The listing builds one solid part. Answer for the finished solid, in the listing's coordinates (mm). Face numbers are marked on the shaded views. A direction names the side the tool comes from. Coordinates: 2 decimals unless noted, no trailing zeros. Order: outer loops, then holes, each group sorted by start corner. A loop starts at its lowest first (then second) coordinate and runs counter-clockwise, first axis right, second up. Notation, with made-up numbers: (-4.5, -17) - (21.5, -17) arc R19 ccw to (21.5, -11) - close; hole circle Ø9 at (-26.5, 15.5). An arc over 180 degrees is marked (long way). Use one line per item in the form item = value. Start each with the question number.
Item 1: Each of these flat-tipped pins is pushed along its axis until it touches: pin 1 Ø4 at (x, y) = (0, 0) entering from +Z; pin 2 Ø4 at (x, y) = (-29, 34) entering from +Z; pin 3 Ø8 at (x, z) = (-15, 7) entering from -Y; pin 4 Ø5 at (x, z) = (8.5, 8) entering from +Y. Where does it stop, or does it pass through?
Item 2: A tool of negligible diameter and unlimited length cuts with its end or side. For the marked faces 1, 2, 3, 4 and 5, from which of +Z, -Z, +X, -X, +Y, -Y can it reach the whole face along a straight path? Write none if from no direction.
Item 3: Section A-A, the plane y = 0 is taken. Count the separate pieces of the cut face and the enclosed holes in it, and give its area (3 significant figures).
Item 4: Section C-C, the plane z = 10 is taken. Write down the section's boundary in (x, y).
Item 5: Consider line 1 along Z through (x, y) = (37.5, 0) (3 decimals); line 2 along Y through (x, z) = (0, 32); line 3 along Y through (x, z) = (0.5, 13). Determine where each line is inside the solid, lowest interval first. Write a range as [from, to].
Item 6: Section D-D, the plane z = 24.5 is taken. Write down the section's boundary in (x, y).
Item 7: Section B-B, the plane y = -39 is taken. Write down the section's boundary in (x, z), and give its area (3 significant figures).
Item 8: The mould has two halves that part along Y. Classify the marked faces 6, 7, 8 and 9: released by +Y, released by -Y, zero draft, split by the parting line, or undercut.
Autodesk Inventor part; units mm, degrees
ref_plane "Work Plane1" through (44.45, 0, 19) normal (1, 0, 0) x (0, 1, 0)
ref_plane "XZ Plane" through (0, 0, 0) normal (0, 1, 0) x (-1, 0, 0)
ref_plane "XY Plane" through (0, 0, 0) normal (0, 0, 1) x (1, 0, 0)
sketch "Sketch1" plane through (0, 0, 0) normal (0, 1, 0) x (-1, 0, 0)
  line L0 (0, 0) -> (0, 38)
  line L1 (-3.5, 30) -> (-15, 30)
  line L2 (-15, 30) -> (-15, 35)
  line L3 (-15, 35) -> (-34.45, 35)
  line L4 (-34.45, 35) -> (-34.45, 0)
  line L5 (-34.45, 0) -> (-44.45, 0)
  line L6 (-44.45, 0) -> (-44.45, 38)
  line L7 (-44.45, 38) -> (-34.5, 38)
  line L8 (-34.5, 38) -> (-34.5, 39)
  line L9 (-34.5, 39) -> (-31.5, 39)
  line L10 (-31.5, 39) -> (-31.5, 38)
  line L11 (-31.5, 38) -> (-12, 38)
  line L12 (-12, 33) -> (-3.5, 33)
  line L13 (-12, 38) -> (-12, 33)
  line L14 (-3.5, 33) -> (-3.5, 30)
  line L15 (-3.5, 33) -> (-3.5, 36)
  line L16 (-3.5, 36) -> (-6, 36)
  line L17 (-6, 36) -> (-6, 33)
  dimension "d5" = 69
  dimension "d6" = 3
  dimension "d7" = 1
  dimension "d8" = 88.9
  dimension "d10" = 3
  dimension "d11" = 5
  dimension "d12" = 30
  dimension "d37" = 10
  dimension "d64" = 38
  dimension "d74" = 7
  dimension "d75" = 24
  dimension "d76" = 3
  dimension "d77" = 2.5
  dimension "d78" = 3
revolve "Revolution1" add sketch "Sketch1" angle 360 about axis through (0, 0, 0) along (0, 0, 1)
ref_plane "Work Plane1" through (44.45, 0, 19) normal (1, 0, 0) x (0, 1, 0)
sketch "Sketch7" plane through (44.45, 0, 19) normal (1, 0, 0) x (0, 1, 0)
  line L0 (34.45, 16) -> (-34.45, 16)
  line L1 (34.45, -19) -> (-34.45, -19)
  line L2 (34.45, 16) -> (-34.45, 16)
  line L3 (0, 16) -> (0, -19) construction
  line L4 (57.5, 28.575) -> (-57.5, 28.575)
  line L5 (-57.5, 28.575) -> (-57.5, -31.575)
  line L6 (-57.5, -31.575) -> (57.5, -31.575)
  line L7 (57.5, -31.575) -> (57.5, 28.575)
  line L8 (57.5, 28.575) -> (-57.5, -31.575) construction
  line L9 (-57.5, 28.575) -> (57.5, -31.575) construction
  point P0 (0, -1.5)
  dimension "d79" = 115
  dimension "d80" = 60.1501
extrude "Extrusion5" cut sketch "Sketch7" against normal blind 4
chamfer "Chamfer1" distance 0.25 angle 45 4 edges at (-44.45, 0, 38) (-34.5, 0, 39) (-31.5, 0, 39) (40.45, 0, 38)
sketch "Sketch8" plane through (40.45, 0, 19) normal (1, 0, 0) x (0, 0, -1)
  circle A0 centre (0.125, 0) radius 12.5
  line L0 (19, 44.45) -> (19, -44.45)
  line L1 (-19, -44.2) -> (-19, 44.2)
  line L2 (19, -18.4282) -> (-18.75, -18.4282)
  point P0 (19, 0)
  point P1 (19, 18.4282)
  point P2 (-19, -18.3739)
  point P3 (-19, 18.3739)
  point P4 (19, 0)
  point P5 (0.125, -18.4282)
  dimension "d44" = 25
extrude "Extrusion6" cut sketch "Sketch8" against normal blind 20
sketch "Sketch10" plane through (40.45, 0, 19) normal (1, 0, 0) x (0, 0, -1)
  circle A0 centre (0.125, 0) radius 12.5
  line L0 (0.125, 0) -> (19, 0)
  line L1 (19, 18.4282) -> (19, -18.4282)
  line L2 (0.125, 0) -> (12.8529, 12.7279)
  point P0 (19, 0)
  dimension "d51" = 18
  dimension "d65" = 45
hole "Hole2" at (40.45, 12.7279, 6.1471) direction (-1, 0, 0) diameter 2.459 depth 4.5 tip angle 118
pattern_circular "Circular Pattern1" count 4 over 360 about axis through (40.45, 0, 18.875) along (-1, 0, 0) of "Hole2"
sketch "Sketch12" plane through (0, 0, 38) normal (0, 0, 1) x (1, 0, 0)
  circle A0 centre (0, 0) radius 41.45
  circle A1 centre (0, 0) radius 44.45
  point P0 (0, 0)
  dimension "d81" = 82.9
  dimension "d82" = 88.9
extrude "Extrusion9" cut sketch "Sketch12" against normal blind 2
properties part number "008" material "Steel, Carbon"
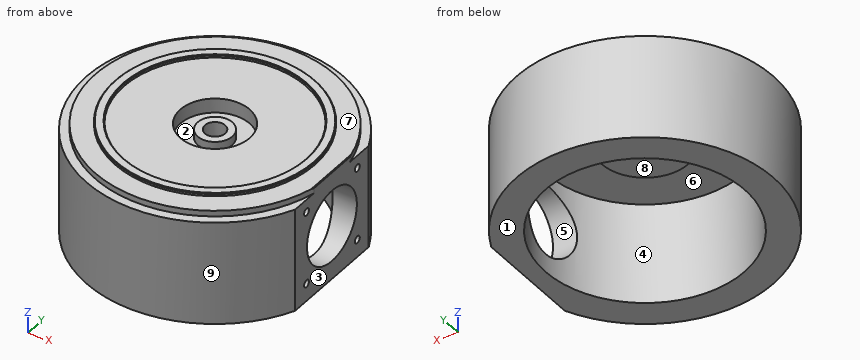
Response:
q1.pin_1 = through
q1.pin_2 = 36
q1.pin_3 = -43.07
q1.pin_4 = 44.04
q2.face_1 = -Z, +X, -X, +Y, -Y
q2.face_2 = +Z
q2.face_3 = +Z, -Z, +X, +Y, -Y
q2.face_4 = -Z
q2.face_5 = +X
q3.separate_pieces = 3
q3.enclosed_holes = 0
q3.area = 689 mm2
q4.outline = (33.31, -8.8) arc R34.45 cw (long way) to (33.31, 8.8) - (40.45, 8.8) - (40.45, 18.43) arc R44.45 ccw (long way) to (40.45, -18.43) - (40.45, -8.8) - close
q5.line_1 = [0, 6.375], [31.375, 38]
q5.line_2 = [-44.45, -34.45], [-15, -3.5], [3.5, 15], [34.45, 44.45]
q5.line_3 = [-44.45, -34.45], [34.45, 44.45]
q6.outline = (32.59, -11.16) arc R34.45 cw (long way) to (32.59, 11.16) - (40.45, 11.16) - (40.45, 18.43) arc R44.45 ccw (long way) to (40.45, -18.43) - (40.45, -11.16) - close
q7.outline = (-21.33, 0) - (21.33, 0) - (21.33, 36) - (14.04, 36) - (14.04, 38) - (-14.04, 38) - (-14.04, 36) - (-21.33, 36) - close
q7.area = 1,590 mm2
q8.face_6 = undercut
q8.face_7 = zero draft
q8.face_8 = undercut
q8.face_9 = split by the parting line
